The figure shows three views and two pictorial views of one solid part (mm, origin at its lowest corner). Answer the questions. A direction names the side the tool comes from. Coordinates: 2 decimals unless noted, no trailing zeros. Order: outer loops, then holes, each group sorted by start corner. A loop starts at its lowest first (then second) coordinate and runs counter-clockwise, first axis right, second up. Notation, with made-up numbers: (41.25, -16) -> (91.25, -16) arc R20 cw to (91.25, 21) -> close; hole circle Ø9 at (63.5, 77). An arc over 180 degrees is marked (long way). Write item = value, one per line. Start each with the question number.
Q1. The part is cut by section A-A, the plane y = 11. Determine the outline of the cut face in (x, z).
Q2. Which of the six approach directions +Z, -Z, +X, -X, +Y, -Y give full straight-line access (tool end or side, diameter ignored) to the marked faces 1, 2, 3, 4 and 5?
Q3. The part is cut by section B-B, the plane x = 54.5. Determine the outline of the cut face in (y, z).
Q4. The part is cut by section D-D, the plane y = 58. Determine the outline of the cut face in (x, z), plus the area to 3 significant figures.
Q5. Straight lines are drawn through the part: L1, parallel to Y at x = 34, z = 119; L2, parallel to Z at x = 89.5, y = 68; L3, parallel to Z at x = 61.5, y = 18. For each, find the intervals that lie inside material, in ascending order. Write a range as from..to.
Q6. Flat-ended cylindrical pins translate along their axes: pin 1 (6 mm diameter, centred on y = 13, z = 130, fed in from +X); pin 2 (1.5 mm diameter, centred on x = 31.5, y = 23, fed in from +Z); pin 3 (10 mm diameter, centred on y = 14.5, z = 22, fed in from -X). Find the tip coordinate at first contact, or state that the pin passes through.
Q7. The part is cut by section C-C, the plane z = 14. Determine the outline of the cut face in (x, y), plus the area to 3 significant figures.
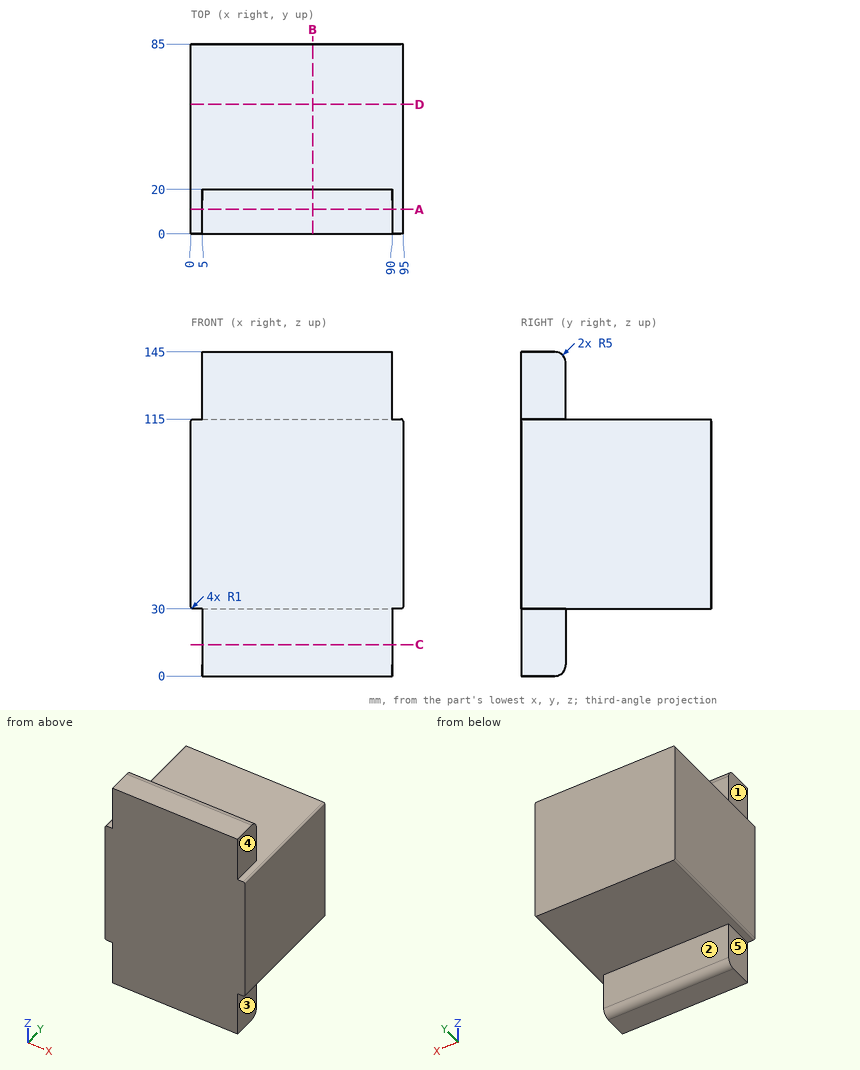
Model answer:
q1.outline = (0, 31) arc R1 ccw to (1, 30) -> (5, 30) -> (5, 0) -> (90, 0) -> (90, 30) -> (94, 30) arc R1 ccw to (95, 31) -> (95, 114) arc R1 ccw to (94, 115) -> (90, 115) -> (90, 145) -> (5, 145) -> (5, 115) -> (1, 115) arc R1 ccw to (0, 114) -> close
q2.face_1 = +Z, -X, +Y, -Y
q2.face_2 = -Z, +X, -X, +Y
q2.face_3 = -Z, +X, +Y, -Y
q2.face_4 = +Z, +X, +Y, -Y
q2.face_5 = -Z, -X, +Y, -Y
q3.outline = (0, 0) -> (15, 0) arc R5 ccw to (20, 5) -> (20, 30) -> (85, 30) -> (85, 115) -> (20, 115) -> (20, 140) arc R5 ccw to (15, 145) -> (0, 145) -> close
q4.outline = (0, 31) arc R1 ccw to (1, 30) -> (94, 30) arc R1 ccw to (95, 31) -> (95, 114) arc R1 ccw to (94, 115) -> (1, 115) arc R1 ccw to (0, 114) -> close
q4.area = 8,070 mm2
q5.L1 = 0..20
q5.L2 = 30..115
q5.L3 = 1..144
q6.pin_1 = 90
q6.pin_2 = 115
q6.pin_3 = 5
q7.outline = (5, 0) -> (90, 0) -> (90, 20) -> (5, 20) -> close
q7.area = 1,700 mm2
